Design review of the part built by this model. Coordinates are the model's own, in mm. A direction names the side the tool comes from. Coordinates: 2 decimals unless noted, no trailing zeros. Order: outer loops, then holes, each group sorted by start corner. A loop starts at its lowest first (then second) coordinate and runs counter-clockwise, first axis right, second up. Notation, with made-up numbers: (-23, 39.25) -> (-8, 39.25) arc R25 cw to (-8, 51.25) -> close; hole circle Ø6 at (28, -36). An arc over 180 degrees is marked (long way). Write item = value, one per line.
```python
from build123d import *

# Parameters (mm, degrees)
SKETCH1_R          = 87.5
BASE_FLANGE1_DEPTH = 6
SKETCH4_W          = 30
SKETCH4_H          = 3
CUT_EXTRUDE1_DEPTH = 10
CIRPATTERN1_COUNT  = 8


# Sheet-metal steps are written as plain solids
with BuildPart() as part:
    # Sketch1 → Base-Flange1 (new body)
    with BuildSketch(Plane(origin=(0, 0, 0), x_dir=(1, 0, 0), z_dir=(0, 1, 0))):
        with Locations(Location((0, 0, 0), (0, 0, 270))):
            Circle(SKETCH1_R)
    extrude(amount=-BASE_FLANGE1_DEPTH)

    # Sketch4 → Cut-Extrude1 (cut)
    with BuildSketch(Plane(origin=(0, 0, 0), x_dir=(1, 0, 0), z_dir=(0, 1, 0))):
        with Locations((-21, 0)):
            Rectangle(SKETCH4_W, SKETCH4_H)
    cut_extrude1 = extrude(amount=-CUT_EXTRUDE1_DEPTH, mode=Mode.SUBTRACT)

    # CirPattern1: Cut-Extrude1 ×8 about axis
    cirpattern1_axis = Axis((0, 0, 0), (0, 1, 0))
    for i in range(1, CIRPATTERN1_COUNT):
        add(cut_extrude1.rotate(cirpattern1_axis, i * 360 / CIRPATTERN1_COUNT), mode=Mode.SUBTRACT)


solid = part.part
```
(1) We need section B-B (z = -13.5). Write out the cut boundary in (x, y), and give its area (3 significant figures).
Report:
outline = (-86.45, -6) -> (-15.62, -6) -> (-15.62, 0) -> (-86.45, 0) -> close; (-11.38, -6) -> (-1.5, -6) -> (-1.5, 0) -> (-11.38, 0) -> close; (1.5, -6) -> (11.38, -6) -> (11.38, 0) -> (1.5, 0) -> close; (15.62, -6) -> (86.45, -6) -> (86.45, 0) -> (15.62, 0) -> close
area = 969 mm²
(2) The part is to be moulded in two halves that separate along X. For faces 1 (the cylindrical face through (86.755, -2.958, -11.391)), 2 (the flat face through (13.94, -2.96, -16.06)), 3 (the flat face through (1, 0, -1)), say which applies: released by +X, released by -X, zero draft, split by the parting line, or undercut.
Report:
face_1 = split by the parting line
face_2 = undercut
face_3 = zero draft
(3) Insertion check: pin 1 (3.5 mm diameter, centred on x = -0.5, y = -2, fed in from -Z); pin 2 (1.8 mm diameter, centred on x = 25, y = -4, fed in from -Z); pin 3 (2 mm diameter, centred on x = -9, y = -2.5, fed in from -Z); pin 4 (2 mm diameter, centred on y = -2, z = -42, fed in from +X). Each pin has a flat end and moves straight along its axis. Give the tip position at first contact, or say it passes through.
Report:
pin_1 = -87.5
pin_2 = -84.12
pin_3 = -87.13
pin_4 = 77.3
(4) We need section A-A (y = -1.45). Give the number of separate pieces and of enclosed holes in the cut face, and give its area (3 significant figures).
Report:
separate_pieces = 1
enclosed_holes = 8
area = 23,300 mm²
(5) We need section C-C (x = -66.5). Write out the cut boundary in (y, z), and give its area (3 significant figures).
Report:
outline = (-6, -56.87) -> (0, -56.87) -> (0, 56.87) -> (-6, 56.87) -> close
area = 682 mm²
(6) For faces 4 (the flat face through (1, -6, -1)), 5 (the flat face through (16.06, -2.96, -13.94)), list the 3-axis set-ups (+Z, -Z, +X, -X, +Y, -Y) from which the entire face can be reached by the end or side of a thin tool; tool diameter is ignored.
Report:
face_4 = +Z, -Z, +X, -X, -Y
face_5 = +Y, -Y
(7) We need section D-D (z = -70.5). Write out the cut boundary in (x, y).
Report:
outline = (-51.83, -6) -> (51.83, -6) -> (51.83, 0) -> (-51.83, 0) -> close
(8) For L1, parallel to X at y = -5.2, z = -11; L2, parallel to X at y = -5.7, z = -19; L3, parallel to Z at x = -10.5, y = -5, list the stretches that pass through material, from the lowest coordinate up.
Report:
L1 = -86.81 to -13.12, -8.88 to -1.5, 1.5 to 8.88, 13.12 to 86.81
L2 = -85.41 to -21.12, -16.88 to -1.5, 1.5 to 16.88, 21.12 to 85.41
L3 = -86.87 to -12.62, -8.38 to -1.5, 1.5 to 8.38, 12.62 to 86.87
